Answer from the drawing. Dimensions are ordinates in mm from the lowest x, y and z of the part. A direction names the side the tool comes from. Round coordinates to 2 decimals unless told otherwise and drop trailing zeros. Order: outer loops, then holes, each group sorted by start corner. A loop starts at its lowest first (then second) coordinate and runs counter-clockwise, first axis right, second up. Notation, with made-up numbers: M 25.25,-5.5 L 60.25,-5.5 A23 cw 60.25,26.5 Z; hole C -20,41 d7. An arc over 180 degrees is marked long. Use one line per item in the form item = value. Start each with the question number.
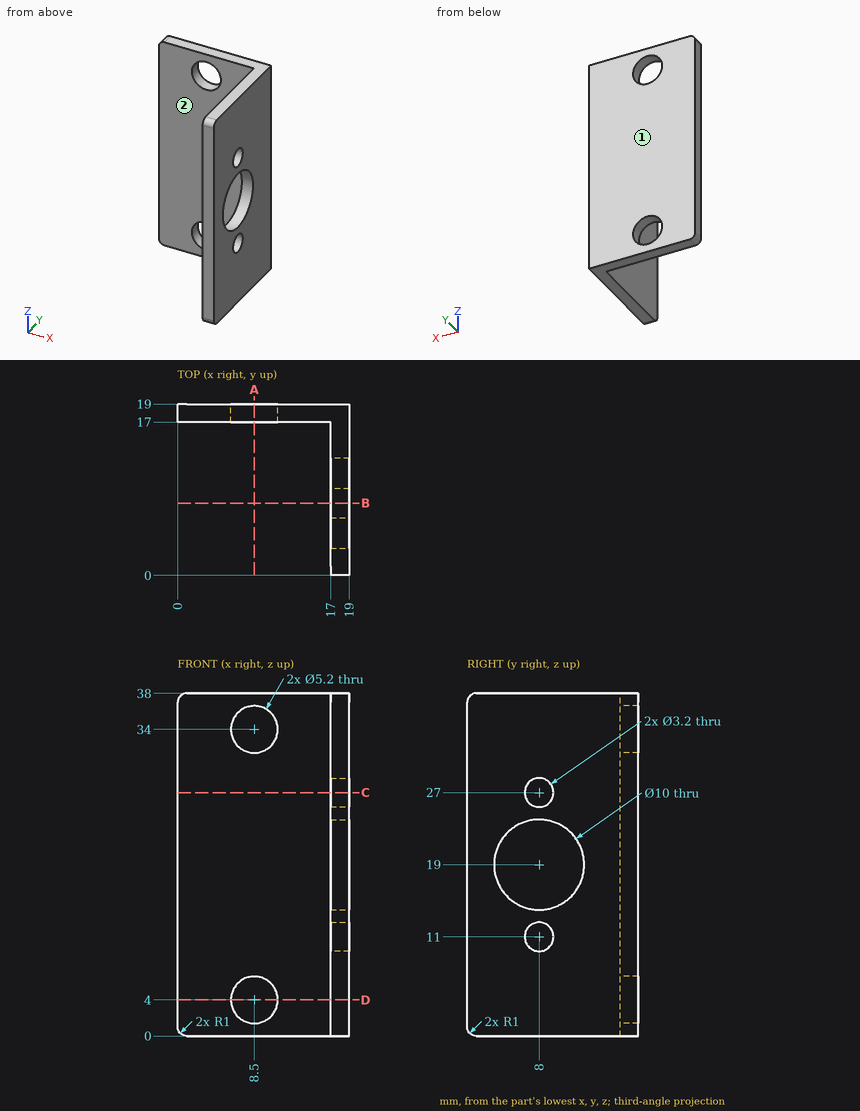
Item 1: Section B-B (y = 8) is taken. Write down the section's boundary in (x, z).
Item 2: Section C-C (z = 27) is taken. Write down the section's boundary in (x, y).
Item 3: A tool of negligible diameter and unlimited length cuts with its end or side. For the marked faces 1 and 2, from which of +Z, -Z, +X, -X, +Y, -Y can it reach the whole face along a straight path? Write none if from no direction.
Item 4: Find the intervals of material crossed by L1, parallel to Z at x = 8.5, y = 17.95; L2, parallel to X at y = 18.25, z = 4; L3, parallel to X at y = 3.25, z = 2.5, in increasing order. Write a range as [from, to].
Item 5: Given P1, Ø8.5, axis at y = 10.5, z = 19.5, coming from the -X side; P2, Ø8.5, axis at x = 6.5, z = 14, coming from the -Y side, each flat-ended and moving along its own axis, determine where each tip first touches the part or whether it passes through.
Item 6: Section A-A (x = 8.5) is taken. Write down the section's boundary in (y, z), and give its area (3 significant figures).
Item 7: Section D-D (z = 4) is taken. Write down the section's boundary in (x, y), and give its area (3 significant figures).
The answers:
q1.outline = M 17,0 L 19,0 L 19,9.4 L 17,9.4 Z; M 17,12.6 L 19,12.6 L 19,14 L 17,14 Z; M 17,24 L 19,24 L 19,25.4 L 17,25.4 Z; M 17,28.6 L 19,28.6 L 19,38 L 17,38 Z
q2.outline = M 0,17 L 17,17 L 17,9.6 L 19,9.6 L 19,19 L 0,19 Z; M 17,0 L 19,0 L 19,6.4 L 17,6.4 Z
q3.face_1 = +Z, -Z, +X, -X, +Y
q3.face_2 = +Z, -Z, -X, -Y
q4.L1 = [0, 1.4], [6.6, 31.4], [36.6, 38]
q4.L2 = [0, 5.9], [11.1, 19]
q4.L3 = [17, 19]
q5.P1 = 17
q5.P2 = 17
q6.outline = M 17,0 L 19,0 L 19,1.4 L 17,1.4 Z; M 17,6.6 L 19,6.6 L 19,31.4 L 17,31.4 Z; M 17,36.6 L 19,36.6 L 19,38 L 17,38 Z
q6.area = 55.2 mm²
q7.outline = M 0,17 L 5.9,17 L 5.9,19 L 0,19 Z; M 11.1,17 L 17,17 L 17,0 L 19,0 L 19,19 L 11.1,19 Z
q7.area = 61.6 mm²
